The figure shows three views and two pictorial views of one solid part (mm, origin at its lowest corner). Answer the questions. Coordinates: 2 decimals unless noted, no trailing zeros. Order: outer loops, then holes, each group sorted by start corner. A loop starts at its lowest first (then second) coordinate and runs counter-clockwise, first axis right, second up. Notation, with made-up numbers: (-23, 24) -> (11, 24) arc R23 ccw to (11, 38) -> close; hole circle Ø7 at (6, -14). An arc over 180 degrees is marked (long way). Return JSON: item names as keys, results as strings.
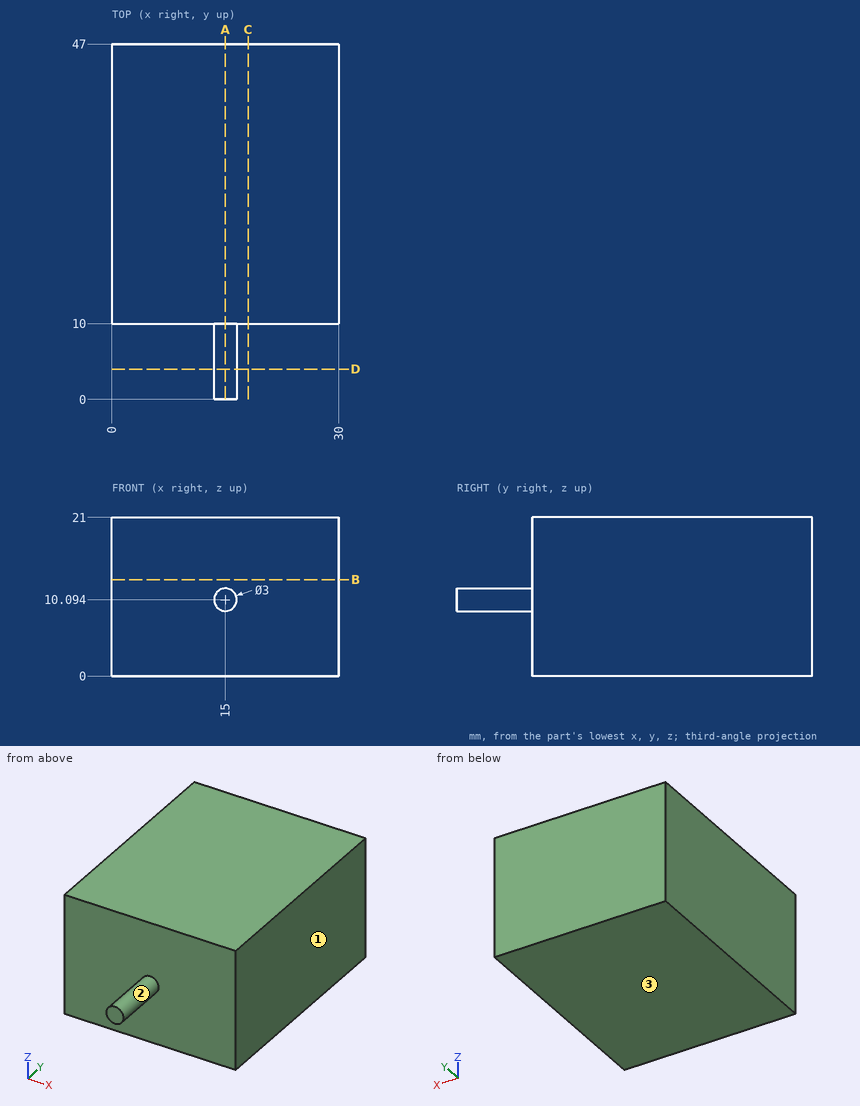
1. The part is cut by section D-D on y = 4. Give the vertices of the cut face in (x, z) (1 decimal).
Answer block:
{"outline": "circle Ø3 at (15, 10.1)"}
2. The part is cut by section A-A on x = 15. Give the vertices of the cut face in (y, z) (1 decimal), and give its area (3 significant figures).
Answer block:
{"outline": "(0, 8.6) -> (10, 8.6) -> (10, 0) -> (47, 0) -> (47, 21) -> (10, 21) -> (10, 11.6) -> (0, 11.6) -> close", "area": "807 mm2"}
3. The part is cut by section B-B on z = 12.75. Give the vertices of the cut face in (x, y), and give its area (3 significant figures).
Answer block:
{"outline": "(0, 10) -> (30, 10) -> (30, 47) -> (0, 47) -> close", "area": "1,110 mm2"}
4. This flat-tipped pin is pushed along its axis until it touches: pin 1 Ø12 at (x, z) = (3.5, 2.5) entering from -Y. Where does it stop, or does it pass through?
Answer block:
{"pin 1": "stops at y = 10"}
5. Determine the mould class of the marked faces 1, 2 and 3 for opening direction X: pulls with the +X half, pulls with the -X half, needs draft (parallel to the pull), parting line crosses it, or undercut.
Answer block:
{"face 1": "pulls with the +X half", "face 2": "parting line crosses it", "face 3": "needs draft"}
6. The part is cut by section C-C on x = 18. Give the vertices of the cut face in (y, z).
Answer block:
{"outline": "(10, 0) -> (47, 0) -> (47, 21) -> (10, 21) -> close"}
7. Consider line 1 (Y direction, x = 2.5, z = 18); line 2 (Z direction, x = 13.75, y = 9.5) (1 decimal); line 3 (X direction, y = 7, z = 11.25) (1 decimal). Determine where each line is inside the solid, lowest interval first. Write a range as from..to.
Answer block:
{"line 1": "y = 10..47", "line 2": "z = 9.3..10.9", "line 3": "x = 14..16"}
